Source: CAD feature listing. Evaluate the final solid. Frame: model axes, mm. Face numbers are marked on the shaded views. Give positions to 0.01 mm unless a question says otherwise; leave off trailing zeros. Order: outer loops, then holes, each group sorted by start corner. A loop starts at its lowest first (then second) coordinate and runs counter-clockwise, first axis right, second up. Notation, with made-up numbers: (43, -14.75) -> (95, -14.75) arc R31 ccw to (95, 22.25) -> close; hole circle Ø1 at (62, 36). An arc over 180 degrees is marked (long way). Use one line per item in the form item = value. Start each with the question number.
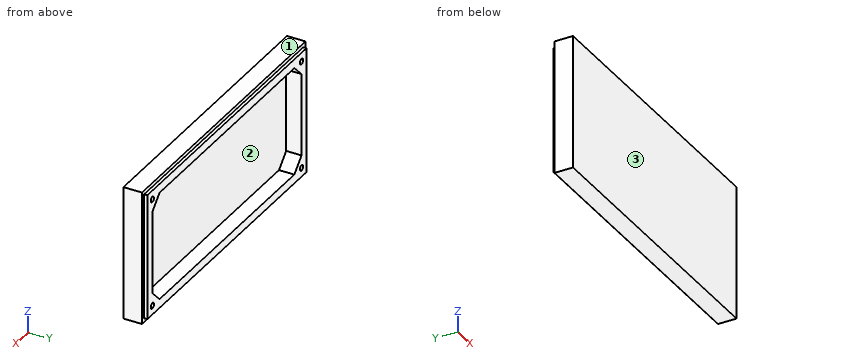
from build123d import *

# Parameters (mm, degrees)
SLABSKETCH_W            = 455
SLABSKETCH_H            = 210
SLAB_DEPTH              = 34
CUT_DEPTH               = 24
DIVOTSKETCH_OUTSIDE_W   = 557.456
DIVOTSKETCH_OUTSIDE_H   = 312.456
DIVOTSKETCH_OUTSIDE_W_2 = 443
DIVOTSKETCH_OUTSIDE_H_2 = 198
DIVOT_DEPTH             = 5
PILOTHOLESSKETCH_R      = 4.4
PILOTHOLES_DEPTH        = 20


with BuildPart() as part:
    # slabSketch → slab (new body)
    with BuildSketch(Plane(origin=(0, 0, 0), x_dir=(1, 0, 0), z_dir=(0, 1, 0))):
        with Locations((227.5, 105)):
            Rectangle(SLABSKETCH_W, SLABSKETCH_H)
    extrude(amount=-SLAB_DEPTH)

    # cutSketch → cut (cut)
    with BuildSketch(Plane(origin=(0, 0, 0), x_dir=(1, 0, 0), z_dir=(0, 1, 0))):
        Polygon((40, 190), (20, 170), (20, 40), (40, 20), (415, 20), (435, 40), (435, 170), (415, 190), align=None)
    extrude(amount=-CUT_DEPTH, mode=Mode.SUBTRACT)

    # divotSketch outside → divot (cut)
    with BuildSketch(Plane(origin=(0, 0, 0), x_dir=(1, 0, 0), z_dir=(0, 1, 0))):
        with Locations((227.5, 105)):
            Rectangle(DIVOTSKETCH_OUTSIDE_W, DIVOTSKETCH_OUTSIDE_H)
        with Locations((227.5, 105)):
            Rectangle(DIVOTSKETCH_OUTSIDE_W_2, DIVOTSKETCH_OUTSIDE_H_2, mode=Mode.SUBTRACT)
    extrude(amount=-DIVOT_DEPTH, mode=Mode.SUBTRACT)

    # pilotholesSketch → pilotholes (cut)
    with BuildSketch(Plane(origin=(0, 0, 0), x_dir=(1, 0, 0), z_dir=(0, 1, 0))):
        with Locations((20, 190)):
            Circle(PILOTHOLESSKETCH_R)
        with Locations((435, 190)):
            Circle(PILOTHOLESSKETCH_R)
        with Locations((435, 20)):
            Circle(PILOTHOLESSKETCH_R)
        with Locations((20, 20)):
            Circle(PILOTHOLESSKETCH_R)
    extrude(amount=-PILOTHOLES_DEPTH, mode=Mode.SUBTRACT)


solid = part.part
1) Pin query (flat end, axial travel): pin 1 (10 mm diameter, centred on x = 344, z = -122, fed in from +Y); pin 2 (2.5 mm diameter, centred on x = 19.5, z = -21, fed in from +Y); pin 3 (4 mm diameter, centred on x = 137, y = -2, fed in from -Z). Return the tip coordinate at first contact, or that it passes through.
2) Cut plane C-C, the plane x = 238. Return the cut outline in (y, z).
3) Draft query along Z for the marked faces 1, 2 and 3. Return one class per face: +Z half, -Z half, draft (parallel to the pull), parting line (faces both ways), or undercut.
4) Cut plane A-A, the plane y = -10. Return the cut outline in (x, z).
5) Cut plane B-B, the plane z = -113. Return the cut outline in (x, y), plus the area to 3 significant figures.
6) Material intervals for probe 1 along X at (y, z) = (-23, -81); probe 2 along Z at (x, y) = (141, -4.5); probe 3 along Z at (x, y) = (194.5, -17.5), sorted ascending.
Output values:
q1.pin_1 = -24
q1.pin_2 = -20
q1.pin_3 = -204
q2.outline = (-34, -210) -> (-5, -210) -> (-5, -204) -> (0, -204) -> (0, -190) -> (-24, -190) -> (-24, -20) -> (0, -20) -> (0, -6) -> (-5, -6) -> (-5, 0) -> (-34, 0) -> close
q3.face_1 = +Z half
q3.face_2 = undercut
q3.face_3 = draft
q4.outline = (0, -210) -> (455, -210) -> (455, 0) -> (0, 0) -> close; hole circle Ø8.8 at (20, -190); hole circle Ø8.8 at (20, -20); hole (20, -170) -> (40, -190) -> (415, -190) -> (435, -170) -> (435, -40) -> (415, -20) -> (40, -20) -> (20, -40) -> close; hole circle Ø8.8 at (435, -190); hole circle Ø8.8 at (435, -20)
q5.outline = (0, -34) -> (455, -34) -> (455, -5) -> (449, -5) -> (449, 0) -> (435, 0) -> (435, -24) -> (20, -24) -> (20, 0) -> (6, 0) -> (6, -5) -> (0, -5) -> close
q5.area = 5,450 mm^2
q6.probe_1 = 0 to 20, 435 to 455
q6.probe_2 = -204 to -190, -20 to -6
q6.probe_3 = -210 to -190, -20 to 0
